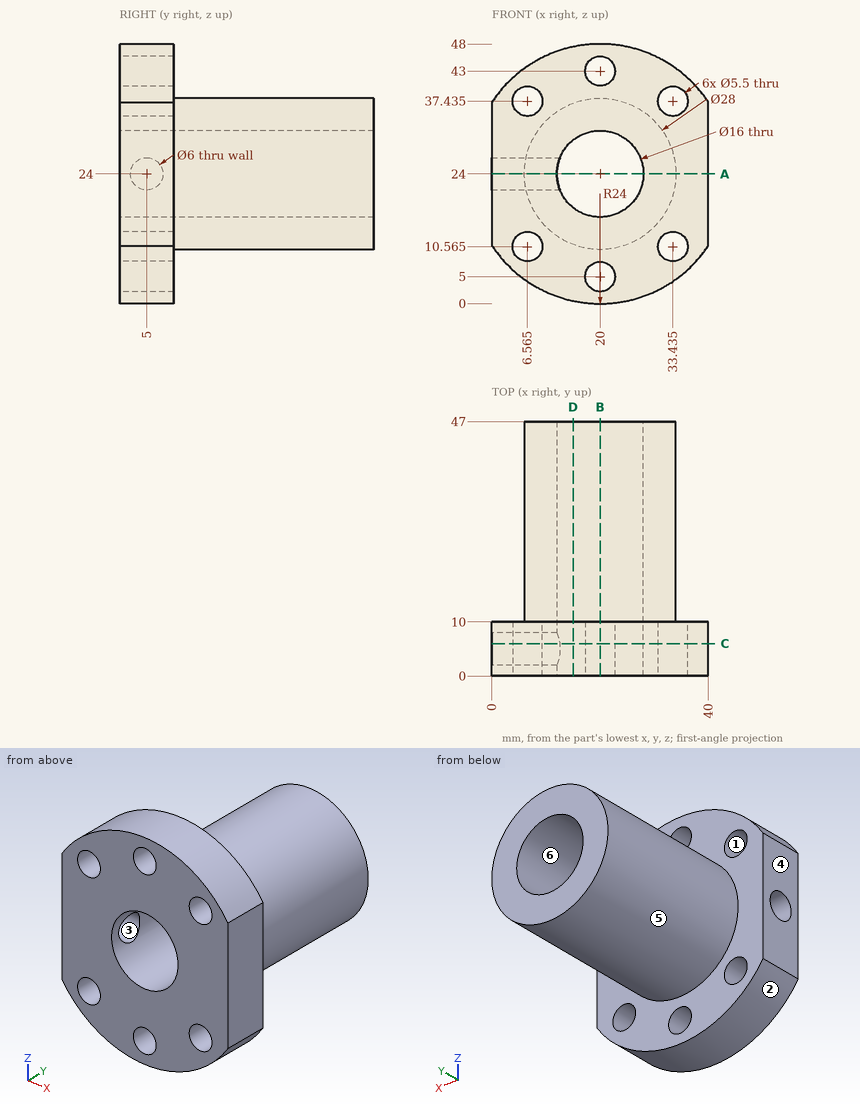
Design review of the part shown in the three views and the two pictorial views. Dimensions are in mm from the part's minimum x, y and z. A direction names the side the tool comes from. Round coordinates to 2 decimals unless told otherwise and drop trailing zeros. Loops run counter-clockwise (first coordinate to the right, second up) from the corner with the lowest first, then second, coordinate; pieces in that order, holes last. Notation, with made-up numbers: M 76.5,50.25 L 134.5,50.25 A13 cw 134.5,72.25 Z; hole C -13,52.25 d8. An arc over 180 degrees is marked long. Answer as a JSON object with one key per item and string values.
Item 1: The part is to be moulded in two halves that separate along X. For the marked faces 1, 2, 3 and 4, say which applies: +X half, -X half, draft (parallel to the pull), parting line (faces both ways), or undercut.
Check sheet entries:
{"face 1": "undercut", "face 2": "parting line", "face 3": "draft", "face 4": "-X half"}
Item 2: We need section C-C, the plane y = 6. State how many separate pieces and enclosed holes the cut face has, and give its area (3 significant figures).
Check sheet entries:
{"separate pieces": "1", "enclosed holes": "6", "area": "1,250 mm2"}
Item 3: We need section B-B, the plane x = 20. State the section outline as (y, z) points.
Check sheet entries:
{"outline": "M 0,0 L 10,0 L 10,2.25 L 0,2.25 Z; M 0,7.75 L 10,7.75 L 10,10 L 47,10 L 47,16 L 0,16 Z; M 0,32 L 47,32 L 47,38 L 10,38 L 10,40.25 L 0,40.25 Z; M 0,45.75 L 10,45.75 L 10,48 L 0,48 Z"}
Item 4: Clearance check with flat-ended pins moving along their axes: P1, Ø8, axis at x = 5.5, y = 6, coming from the +Z side; P2, Ø10, axis at x = 27.5, y = 13, coming from the +Z side; P3, Ø6, axis at x = 30.5, y = 38.5, coming from the +Z side; P4, Ø3.5, axis at x = 33.44, z = 37.44, coming from the -Y side. State where each tip first meets the part, or that it passes through.
Check sheet entries:
{"P1": "z = 45.58", "P2": "z = 47.74", "P3": "z = 35.82", "P4": "through"}
Item 5: We need section A-A, the plane z = 24. State the section outline as (x, y) points.
Check sheet entries:
{"outline": "M 0,0 L 12,0 L 12,2 L 0,2 Z; M 0,8 L 12,8 L 12,47 L 6,47 L 6,10 L 0,10 Z; M 28,0 L 40,0 L 40,10 L 34,10 L 34,47 L 28,47 Z"}
Item 6: We need section D-D, the plane x = 15. State the section outline as (y, z) points (3 decimals), and give its area (3 significant figures).
Check sheet entries:
{"outline": "M 0,0.527 L 10,0.527 L 10,10.923 L 47,10.923 L 47,17.755 L 0,17.755 Z; M 0,30.245 L 47,30.245 L 47,37.077 L 10,37.077 L 10,47.473 L 0,47.473 Z", "area": "850 mm2"}
Item 7: Tool access review of the marked faces 5 and 6: name each direction out of +Z, -Z, +X, -X, +Y, -Y from which nothing blocks a thin tool from reaching the whole face with its end or side.
Check sheet entries:
{"face 5": "+Y", "face 6": "+Y, -Y"}
Item 8: For line 1 along X through (y, z) = (11, 24); line 2 along Z through (x, y) = (20, 27); line 3 along Y through (x, z) = (34.5, 22.5), list the stretches that pass through material, from the lowest coordinate up.
Check sheet entries:
{"line 1": "6 to 12, 28 to 34", "line 2": "10 to 16, 32 to 38", "line 3": "0 to 10"}
